For this review, take the finished solid that the model builds, in its own axes (mm). Coordinates: 2 decimals unless noted, no trailing zeros. Loops run counter-clockwise (first coordinate to the right, second up) from the corner with the lowest first, then second, coordinate; pieces in that order, holes last. Notation, with made-up numbers: (6, 48) - (38, 48) arc R25 ccw to (38, 71) - close; hole circle Ø2 at (-12, 42.5). An arc over 180 degrees is marked (long way). One line per item, written item: value. Start each with the question number.
1. Take a section at A-A, the plane z = 157.5. State the section outline as (x, y) points, and give its area (3 significant figures).
2. Take a section at B-B, the plane z = 53.5. State the section outline as (x, y) points, and give its area (3 significant figures).
3. To check wall thickness, follow line 1 (Y direction, x = 0, z = 34); line 2 (X direction, y = -0.75, z = 173); line 3 (Y direction, x = -1, z = 116.5). State the ranges of each line that lie inside material, in increasing order. Write a range as from..to.
4. Insertion check: pin 1 (4 mm diameter, centred on y = -2.5, z = 218.5, fed in from +X); pin 2 (2 mm diameter, centred on y = -1.5, z = 380, fed in from -X); pin 3 (1.5 mm diameter, centred on x = 2.5, y = -1, fed in from -Z); pin 4 (6 mm diameter, centred on x = 3.5, y = -2, fed in from +Z). Each pin has a flat end and moves straight along its axis. Give the tip position at first contact, or say it passes through.
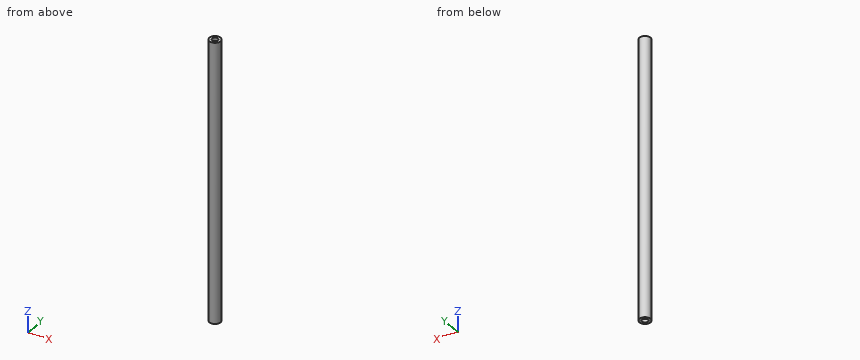
Autodesk Inventor part; units mm, degrees
ref_plane "YZ Plane" through (0, 0, 0) normal (1, 0, 0) x (0, 1, 0)
ref_plane "XZ Plane" through (0, 0, 0) normal (0, 1, 0) x (-1, 0, 0)
ref_plane "XY Plane" through (0, 0, 0) normal (0, 0, 1) x (1, 0, 0)
sketch "Sketch1" plane through (0, 0, 0) normal (0, 0, 1) x (1, 0, 0)
  circle A0 centre (0, 0) radius 9.5
  dimension "d0" = 19
extrude "Extrusion1" add sketch "Sketch1" along normal blind 470
hole "Hole1" at (0, 0, 470) direction (0, 0, -1) diameter 10 depth 70 tip angle 118
hole "Hole2" at (0, 0, 0) direction (0, 0, 1) diameter 10 depth 70 tip angle 118
properties part number "Barra-garfo" material "Aluminium AW-7020"
Solutions:
1. outline: circle Ø19 at (0, 0)
1. area: 284 mm2
2. outline: circle Ø19 at (0, 0); hole circle Ø10 at (0, 0)
2. area: 205 mm2
3. line 1: -9.5..-5, 5..9.5
3. line 2: -9.47..9.47
3. line 3: -9.45..9.45
4. pin 1: x = 9.49
4. pin 2: x = -9.49
4. pin 3: z = 70.94
4. pin 4: z = 470
